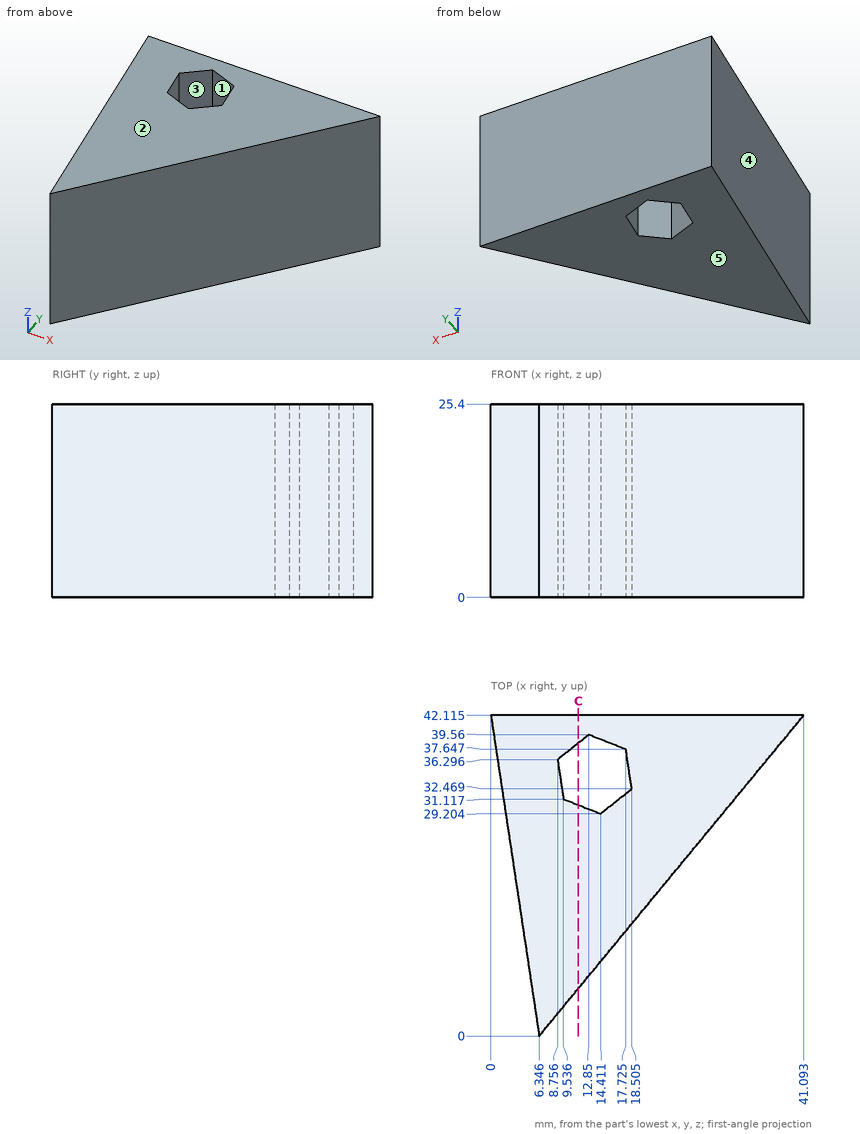
Answer from the drawing. Dimensions are ordinates in mm from the lowest x, y and z of the part. A direction names the side the tool comes from. Give positions to 0.01 mm unless a question says otherwise; leave off trailing zeros. Order: outer loops, then holes, each group sorted by start corner. A loop starts at its lowest first (then second) coordinate and runs counter-clockwise, first axis right, second up. Notation, with made-up numbers: (82, 39) -> (124, 39) arc R29 ccw to (124, 63) -> close; hole circle Ø10 at (13.25, 63). An arc over 180 degrees is marked (long way). One line per item, written item: value. Start each with the question number.
(1) Straight lines are drawn through the part: L1, parallel to Y at x = 15, z = 12 (1 decimal); L2, parallel to Y at x = 24, z = 23 (1 decimal); L3, parallel to X at y = 5.5, z = 22.5 (1 decimal). For each, find the intervals that lie inside material, in ascending order.
(2) For a pull along X with two mould halves and no side action, classify the marked faces 3, 4 and 5 as released by +X, released by -X, zero draft, split by the parting line, or undercut.
(3) Flat-ended cylindrical pins translate along their axes: P1, Ø1.5, axis at x = 25.5, y = 34.5, coming from the -Z side; P2, Ø1, axis at y = 23.5, z = 20.5, coming from the -X side; P3, Ø1.5, axis at y = 21, z = 8.5, coming from the -X side; P4, Ø1.5, axis at y = 9.5, z = 18, coming from the +X side. Find the tip coordinate at first contact, or state that the pin passes through.
(4) The part is cut by section C-C (x = 11.5). Determine the outline of the cut face in (y, z) (1 decimal), and give its area (3 significant figures).
(5) A tool of negligible diameter and unlimited length cuts with its end or side. For the marked faces 1 and 2, from which of +Z, -Z, +X, -X, +Y, -Y can it reach the whole face along a straight path? Write none if from no direction.
Taken from the geometry:
1. L1: 10.5 to 29.7, 38.7 to 42.1
1. L2: 21.4 to 42.1
1. L3: 5.5 to 10.9
2. face 3: undercut
2. face 4: released by -X
2. face 5: zero draft
3. P1: z = 0
3. P2: x = 2.73
3. P3: x = 3.07
3. P4: x = 14.8
4. outline: (6.2, 0) -> (30.3, 0) -> (30.3, 25.4) -> (6.2, 25.4) -> close; (38.5, 0) -> (42.1, 0) -> (42.1, 25.4) -> (38.5, 25.4) -> close
4. area: 704 mm^2
5. face 1: +Z, -Z
5. face 2: +Z, +X, -X, +Y, -Y
